from build123d import *

# Parameters (mm, degrees)
SKETCH2_W = 2.75
SKETCH2_H = 1
FILLET1_R = 0.75
FILLET2_R = 0.25


with BuildPart() as part:
    # Sketch1 → Revolve1 (revolve)
    with BuildSketch(Plane.XY, mode=Mode.PRIVATE) as revolve1_sk:
        Polygon((0, 0), (-7.25, 0), (-7.25, -49), (-6.33564091, -49), (-3.5, -49.5), (0, -49.5), align=None)
    revolve(revolve1_sk.sketch.rotate(Axis((0, 0, 0), (0, -1, 0)), 270), axis=Axis((0, 0, 0), (0, -1, 0)))

    # Sketch2 → Revolve2 (revolve)
    with BuildSketch(Plane.XY, mode=Mode.PRIVATE) as revolve2_sk:
        with Locations((-1.375, 0.5)):
            Rectangle(SKETCH2_W, SKETCH2_H)
    revolve(revolve2_sk.sketch.rotate(Axis((0, 0, 0), (0, 1, 0)), 270), axis=Axis((0, 0, 0), (0, 1, 0)))

    # Fillet1
    fillet1_edges = [part.edges().sort_by_distance(p)[0] for p in [
        (0, -49, -7.25),
        (0, 0, -7.25),
    ]]
    fillet(fillet1_edges, radius=FILLET1_R)

    # Fillet2
    fillet2_edges = [part.edges().sort_by_distance(p)[0] for p in [
        (0, 1, 2.75),
    ]]
    fillet(fillet2_edges, radius=FILLET2_R)


solid = part.part
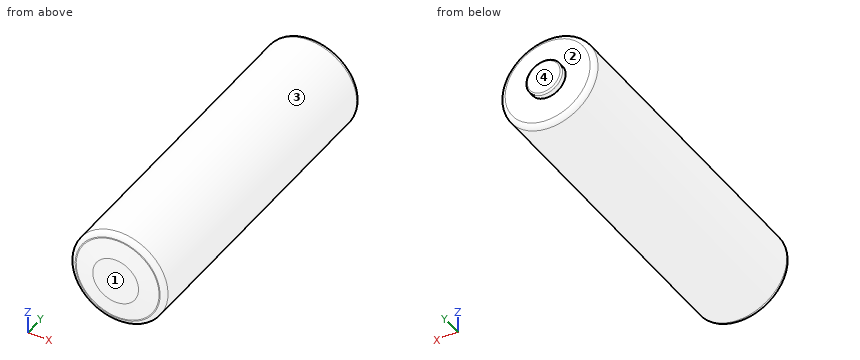
Part model, mm, in its own coordinate system. Face numbers are marked on the shaded views. A direction names the side the tool comes from. Round coordinates to 2 decimals unless told otherwise and drop trailing zeros. Write each loop counter-clockwise with the first axis right and the second up, starting at its lowest first coordinate (ties: lowest second). Pieces come first, ordered by that corner, then holes. Notation, with made-up numbers: M 69.25,-22.75 L 127.25,-22.75 A5 cw 127.25,-14.75 Z; hole C 49,48.25 d1. An arc over 180 degrees is marked long. Return JSON: item names as keys, results as strings. Group by question number.
(1) Which spindle directions (+Z, -Z, +X, -X, +Y, -Y) get a long thin tool onto all of the face, cutting with end or side? Do the marked faces 1 and 2. Say none if no direction does.
(2) Pin check, flat tips, straight feed: pin 1 Ø2 at (x, y) = (3, -35) entering from +Z; pin 2 Ø6 at (y, z) = (-32, -3.5) entering from -X. Stop position of each tip, or through.
(3) Saw through at B-B on z = 0. Write the cut outline in (x, y), then the cut area to 3 significant figures.
(4) Saw through at A-A on x = 0. Write the cut outline in (y, z), then the cut area to 3 significant figures.
(5) Drill centre lines: probe 1 along Y at (x, z) = (4.75, 4.25); probe 2 along X at (y, z) = (-38.5, 0.25); probe 3 along Y at (x, z) = (-1.5, -4.25). Where is each one in solid material? Low to high.
(6) Two-plate mould, pull along Z, no slides. Class the marked faces 3 and 4: +Z half, -Z half, draft (parallel to the pull), parting line (faces both ways), or undercut.
(7) Saw through at C-C on y = -39.5. Write the cut outline in (x, z).
Returned:
{
 "1": {"face 1": "+Z, -Z, +X, -X, -Y", "face 2": "+Y"},
 "2": {"pin 1": "z = 6.97", "pin 2": "x = -7.23"},
 "3": {"outline": "M -7.25,-48.25 A0.75 ccw -6.5,-49 L -6.34,-49 L -3.5,-49.5 L 3.5,-49.5 L 6.34,-49 L 6.5,-49 A0.75 ccw 7.25,-48.25 L 7.25,-0.75 A0.75 ccw 6.5,0 L 2.75,0 L 2.75,0.75 A0.25 ccw 2.5,1 L -2.5,1 A0.25 ccw -2.75,0.75 L -2.75,0 L -6.5,0 A0.75 ccw -7.25,-0.75 Z", "area": "720 mm²"},
 "4": {"outline": "M -49.5,-3.5 L -49,-6.34 L -49,-6.5 A0.75 ccw -48.25,-7.25 L -0.75,-7.25 A0.75 ccw 0,-6.5 L 0,-2.75 L 0.75,-2.75 A0.25 ccw 1,-2.5 L 1,2.5 A0.25 ccw 0.75,2.75 L 0,2.75 L 0,6.5 A0.75 ccw -0.75,7.25 L -48.25,7.25 A0.75 ccw -49,6.5 L -49,6.34 L -49.5,3.5 Z", "area": "720 mm²"},
 "5": {"probe 1": "-49 to 0", "probe 2": "-7.25 to 7.25", "probe 3": "-49.32 to 0"},
 "6": {"face 3": "parting line", "face 4": "draft"},
 "7": {"outline": "C 0,0 d14.5"}
}
